The drawing under review shows one solid part. Ordinate dimensions are in mm from its lowest x, y, z. A direction names the side the tool comes from. Round coordinates to 2 decimals unless told otherwise and drop trailing zeros. Order: outer loops, then holes, each group sorted by start corner. A loop starts at its lowest first (then second) coordinate and runs counter-clockwise, first axis right, second up. Notation, with made-up numbers: M 39.5,71 L 88.5,71 A31 ccw 88.5,103 Z; hole C -2.5,16 d7. An arc over 180 degrees is marked long. Answer as a JSON object with one key per item and string values.
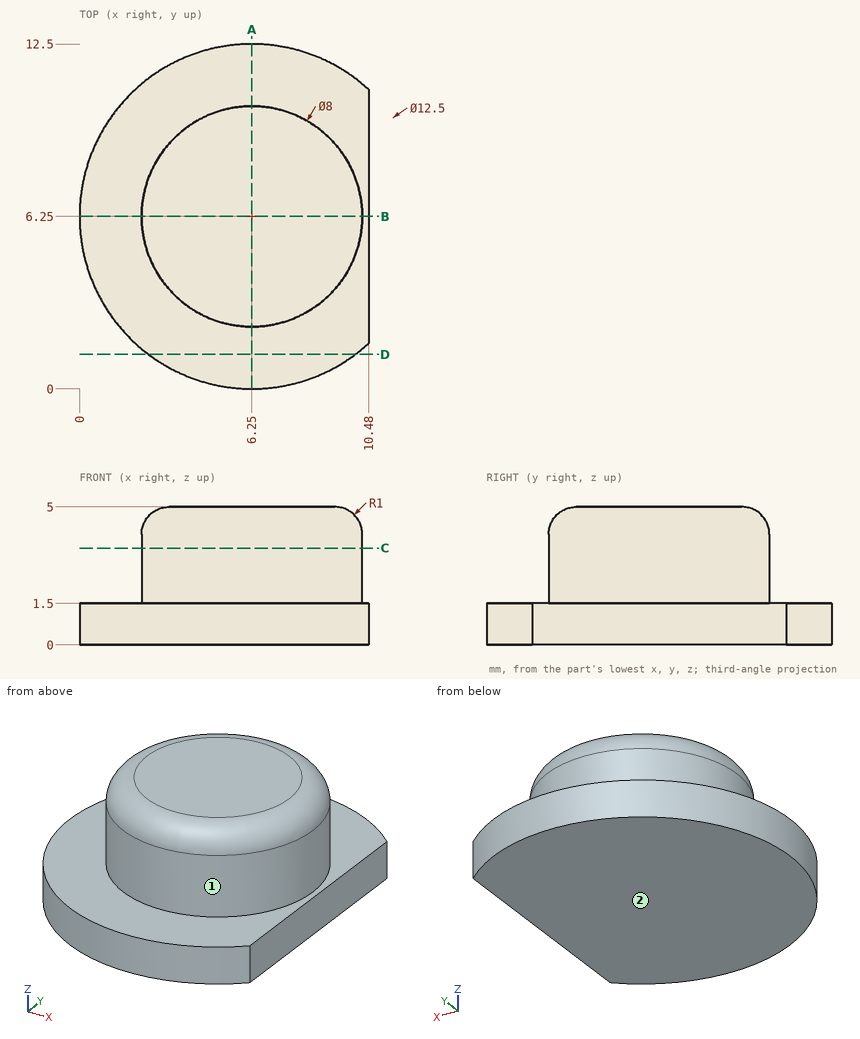
1) Machinability: for the marked faces 1 and 2, which of the approach directions +Z, -Z, +X, -X, +Y, -Y give a long, thin tool a straight path to every point of the face, cutting with its end or side? Answer none if there is none.
Geometry check:
{"face 1": "+Z", "face 2": "-Z, +X, -X, +Y, -Y"}
2) Add section B-B on y = 6.25. State the section outline as (x, z) points, and give its area (3 significant figures).
Geometry check:
{"outline": "M 0,0 L 10.48,0 L 10.48,1.5 L 10.25,1.5 L 10.25,4 A1 ccw 9.25,5 L 3.25,5 A1 ccw 2.25,4 L 2.25,1.5 L 0,1.5 Z", "area": "43.3 mm²"}
3) For L1, parallel to Z at x = 4, y = 11.5; L2, parallel to X at y = 3.5, z = 3.15; L3, parallel to Y at x = 9.25, z = 1.2, list the stretches that pass through material, from the lowest coordinate up.
Geometry check:
{"L1": "z = 0 to 1.5", "L2": "x = 3.35 to 9.15", "L3": "y = 0.77 to 11.73"}
4) Add section A-A on x = 6.25. State the section outline as (y, z) points.
Geometry check:
{"outline": "M 0,0 L 12.5,0 L 12.5,1.5 L 10.25,1.5 L 10.25,4 A1 ccw 9.25,5 L 3.25,5 A1 ccw 2.25,4 L 2.25,1.5 L 0,1.5 Z"}
5) Insertion check: P1, Ø1.5, axis at x = 2.5, z = 1.5, coming from the +Y side; P2, Ø2, axis at x = 5.5, z = 4, coming from the +Y side; P3, Ø1, axis at x = 8, z = 3, coming from the -Y side. Each pin has a flat end and moves straight along its axis. Give the tip position at first contact, or say it passes through.
Geometry check:
{"P1": "stops at y = 11.73", "P2": "stops at y = 10.25", "P3": "stops at y = 2.45"}
6) Add section D-D on y = 1.25. State the section outline as (x, z) points.
Geometry check:
{"outline": "M 2.5,0 L 10,0 L 10,1.5 L 2.5,1.5 Z"}
7) Add section C-C on z = 3.5. State the section outline as (x, y) points, and give its area (3 significant figures).
Geometry check:
{"outline": "C 6.25,6.25 d8", "area": "50.3 mm²"}
